Geometry: final body of the model. Coordinates: model frame, mm. Face numbers are marked on the shaded views. A direction names the side the tool comes from. Give positions to 0.01 mm unless a question says otherwise; leave off trailing zeros. Write each loop counter-clockwise with the first axis right and the second up, starting at its lowest first coordinate (ties: lowest second). Pieces come first, ordered by that corner, then holes.
Q1. Pin query (flat end, axial travel): pin 1 Ø4 at (x, z) = (2.5, 0.5) entering from -Y; pin 2 Ø5 at (x, z) = (1.5, -30) entering from -Y; pin 3 Ø6 at (y, z) = (8, -13) entering from +X; pin 4 Ø10 at (x, y) = (2, 5.5) entering from -Z. Return the tip coordinate at first contact, or that it passes through.
Q2. Section B-B (y = 7). Return the cut outline in (x, z) (3 decimals).
Q3. Line query: line 1 (Z direction, x = 7.75, y = -0.25) (3 decimals); line 2 (X direction, y = 0, z = -26.5); line 3 (Z direction, x = 2, y = 3.5). Output: solid intervals per line, ascending.
Q4. Reachability of the marked faces 1, 2 and 3 from +Z, -Z, +X, -X, +Y, -Y: full face, straight path, thin tool, end or side. Return the list, or none.
Q5. Mould query, pull axis Y, two halves, no side actions, for the marked faces 4, 5 and 6. Classes: +Y half, -Y half, draft (parallel to the pull), parting line (faces both ways), or undercut.
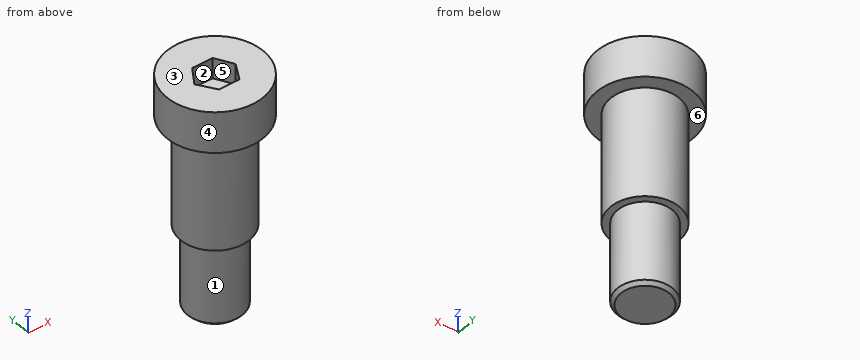
Solid Edge part; units mm, degrees
sketch "Sketch1" plane through (0, 0, 0) normal (0, 0, 1) x (1, 0, 0)
  circle A0 centre (0, 0) radius 11.1125
extrude "Protrusion1" add sketch "Sketch1" along normal blind 9.525
sketch "Sketch2" plane through (0, 0, 0) normal (0, 0, -1) x (0, 1, 0)
  circle A0 centre (0, 0) radius 7.9375
extrude "Protrusion2" add sketch "Sketch2" along normal blind 25.4
sketch "Sketch3" plane through (0, 0, -25.4) normal (0, 0, -1) x (0, 1, 0)
  circle A0 centre (0, 0) radius 6.35
extrude "Protrusion3" add sketch "Sketch3" along normal blind 19.05
sketch "Sketch4" plane through (0, 0, 9.525) normal (0, 0, 1) x (0, 1, 0)
  line L0 (-3.9624, 2.1791) -> (0, 4.7782)
  line L1 (-3.9624, -2.5597) -> (-3.9624, 2.1791)
  line L2 (-3.9624, -2.5597) -> (0, -4.7782)
  line L3 (3.9624, -2.5597) -> (0, -4.7782)
  line L4 (3.9624, -2.5597) -> (3.9624, 2.1791)
  line L5 (3.9624, 2.1791) -> (0, 4.7782)
extrude "Cutout1" cut sketch "Sketch4" against normal blind 4.7625
chamfer "Chamfer1" distance 0.7874 angle 45 1 edges at (0, -6.35, -44.45)
properties part number "24104361"
Computed:
1. pin 1: stops at y = -11.1
1. pin 2: stops at y = -6.35
1. pin 3: stops at x = 6.16
1. pin 4: stops at z = -44.45
2. outline: (-8.631, 0) - (-3.742, 0) - (-3.742, -25.4) - (3.742, -25.4) - (3.742, 0) - (8.631, 0) - (8.631, 9.525) - (-8.631, 9.525) - close
3. line 1: z = -25.4 to 9.525
3. line 2: x = -6.35 to 6.35
3. line 3: z = -44.45 to 4.76
4. face 1: -Z
4. face 2: +Z
4. face 3: +Z, +X, -X, +Y, -Y
5. face 4: parting line
5. face 5: undercut
5. face 6: draft
